Job drawing, mm, ordinate dimensions from the low corner. One solid piece. A direction names the side the tool comes from. Round coordinates to 2 decimals unless told otherwise and drop trailing zeros. Write each loop counter-clockwise with the first axis right and the second up, starting at its lowest first coordinate (ties: lowest second). Pieces come first, ordered by that corner, then holes.
1) Flat gauge pins, fed straight in: pin 1 (5 mm diameter, centred on x = 17.54, y = 37.5, fed in from +Z); pin 2 (12 mm diameter, centred on x = 53, z = 11, fed in from -Y); pin 3 (3 mm diameter, centred on x = 6.77, y = 6.77, fed in from +Z); pin 4 (6 mm diameter, centred on y = 46, z = 12, fed in from +X). Where does each tip first touch, or does it go through?
2) Drill centre lines: L1, parallel to Y at x = 17.5, z = 19.5; L2, parallel to X at y = 37, z = 24 (1 decimal); L3, parallel to X at y = 31, z = 7 (1 decimal). Where is each one in solid material? Low to high.
3) Which spindle directions (+Z, -Z, +X, -X, +Y, -Y) get a long thin tool onto all of the face, cutting with end or side? Do the marked faces 5, 6, 7 and 8. Say none if no direction does.
4) Saw through at D-D on y = 16. Write the cut outline in (x, z) (1 decimal), and give its area (3 significant figures).
5) Saw through at C-C on z = 12. Count the separate pieces of the cut face and the enclosed holes in it.
6) Pull direction X, two halves, no side cores. Call the marked faces 1, 2, 3 and 4: +X half, -X half, draft (parallel to the pull), parting line (faces both ways), or undercut.
7) Saw through at A-A on y = 37.5. Write the cut outline in (x, z) (1 decimal).
8) Saw through at B-B on x = 7. Write the cut outline in (y, z) (1 decimal).
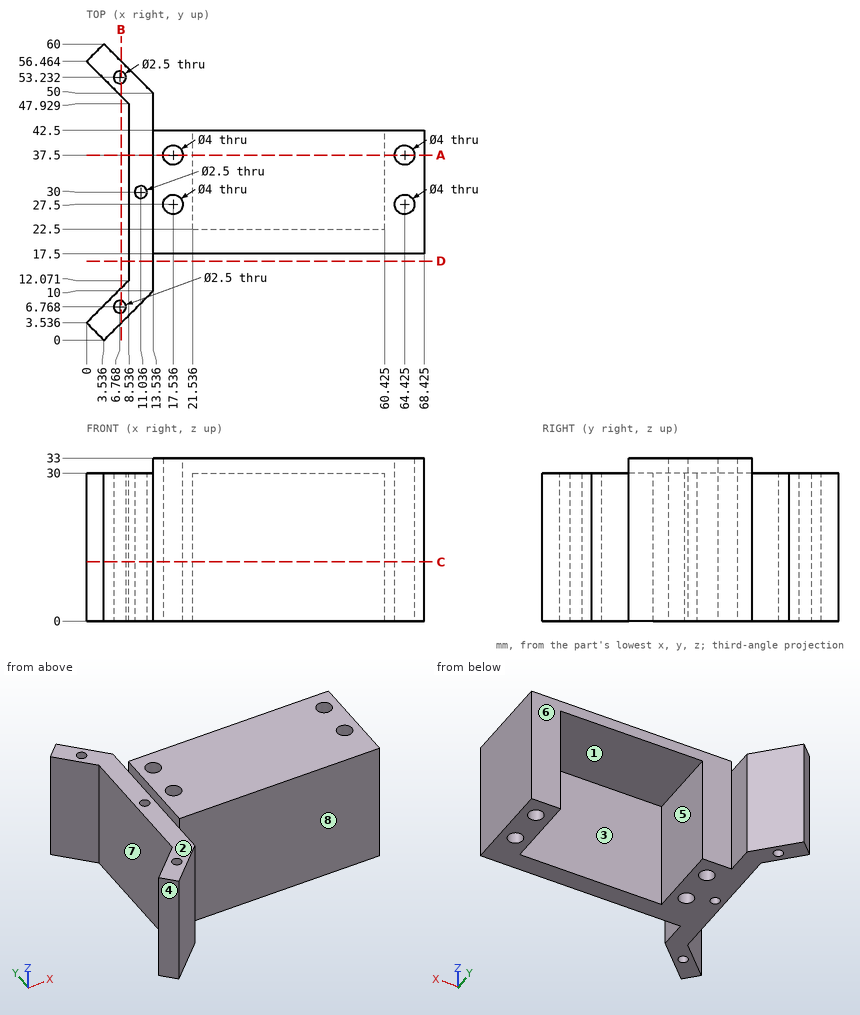
Completed:
1. pin 1: stops at z = 33
1. pin 2: stops at y = 17.5
1. pin 3: stops at z = 30
1. pin 4: stops at x = 13.54
2. L1: y = 17.5 to 25.5, 29.5 to 35.5, 39.5 to 42.5
2. L2: x = 8.5 to 15.6, 19.5 to 21.5, 60.4 to 62.5, 66.4 to 68.4
2. L3: x = 8.5 to 10.3, 11.8 to 21.5, 60.4 to 68.4
3. face 5: -Z, +Y
3. face 6: +Z, -Z, +X, +Y
3. face 7: +Z, -Z, -X
3. face 8: +Z, -Z, +X, -Y
4. outline: (8.5, 0) - (13.5, 0) - (13.5, 30) - (8.5, 30) - close
4. area: 150 mm2
5. separate pieces: 1
5. enclosed holes: 7
6. face 1: undercut
6. face 2: draft
6. face 3: undercut
6. face 4: -X half
7. outline: (8.5, 0) - (15.5, 0) - (15.5, 33) - (13.5, 33) - (13.5, 30) - (8.5, 30) - close; (19.5, 0) - (21.5, 0) - (21.5, 30) - (60.4, 30) - (60.4, 0) - (62.4, 0) - (62.4, 33) - (19.5, 33) - close; (66.4, 0) - (68.4, 0) - (68.4, 33) - (66.4, 33) - close
8. outline: (3.5, 0) - (5.5, 0) - (5.5, 30) - (3.5, 30) - close; (8, 0) - (10.5, 0) - (10.5, 30) - (8, 30) - close; (49.5, 0) - (52, 0) - (52, 30) - (49.5, 30) - close; (54.5, 0) - (56.5, 0) - (56.5, 30) - (54.5, 30) - close
